Part model, mm, in its own coordinate system. A direction names the side the tool comes from. Give positions to 0.01 mm unless a question says otherwise; leave off trailing zeros. Write each loop counter-clockwise with the first axis right and the second up, starting at its lowest first coordinate (ties: lowest second). Pieces come first, ordered by that corner, then holes. Notation, with made-up numbers: M -9,70.5 L 41,70.5 A21 cw 41,81.5 Z; hole C 88,-14 d11. An arc over 180 degrees is marked long. Use CSV: the item, a comma, the result in double quotes. Start each with the question number.
1. Band-saw the part on D-D, the plane y = 63.5. List the corners of the cut face in (x, z).
2. Band-saw the part on C-C, the plane y = 74.5. List the corners of the cut face in (x, z), then the cut area to 3 significant figures.
3. Band-saw the part on B-B, the plane z = 37. List the corners of the cut face in (x, y).
4. Band-saw the part on A-A, the plane x = -37. List the corners of the cut face in (y, z), then the cut area to 3 significant figures.
5. Drop flat-ended pins along their axis: pin 1 Ø4 at (y, z) = (22.5, -35) entering from -X; pin 2 Ø3 at (x, y) = (-44.33, 38.65) entering from +Z; pin 3 Ø20 at (x, y) = (-61.65, 48.65) entering from -Z; pin 4 Ø1.5 at (x, z) = (21, 10) entering from -Y. Give the stop position or say it passes through.
6. 3-axis set-ups, long thin cutter, end or side, ignore diameter. For faces 5 (the face through (-22, 41, 1)), 6 (the face through (-52, 41, 6)), 7 (the face through (-56.574, 38.891, 7.014)): which of +Z, -Z, +X, -X, +Y, -Y reach the whole face in a straight line?
7. Drill centre lines: line 1 along Z through (x, y) = (10, 0.95) (3 decimals); line 2 along X through (y, z) = (0.9, -22) (3 decimals); line 3 along X through (y, z) = (48.65, -38.9). Where is each one in solid material? Low to high. Write a range as from..to.
8. Mould opens along Z. For faces 1 (the face through (-52, 48, -39.5)), 2 (the face through (0, 0, -1)), 3 (the face through (-52, 41, 8)), 4 (the face through (-52, 48, -37.5)) say: pulls with the +Z half, pulls with the -Z half, needs draft (parallel to the pull), parting line crosses it, or undercut.
from build123d import *

# Parameters (mm, degrees)
SKETCH_1_W                   = 50
SKETCH_1_H                   = 100
EXTRUDE_1_DEPTH              = 2
SKETCH_2_W                   = 3
SKETCH_2_H                   = 100
EXTRUDE_2_DEPTH              = 80
SKETCH_3_W                   = 2
SKETCH_3_H                   = 66.7
EXTRUDE_3_DEPTH              = 70
CUT_EXTRUDE_4_REACH          = 162.465
SKETCH_8_W                   = 2
SKETCH_8_H                   = 66.7
EXTRUDE_4_DEPTH              = 70
CUT_EXTRUDE_5_REACH          = 140.25
HOLE_WIZARD_M3_1_D           = 2.5
HOLE_WIZARD_M3_1_DEPTH       = 2
HOLE_WIZARD_M3_1_CSINK_D     = 3.05
HOLE_WIZARD_M3_1_CSINK_ANGLE = 90
FILLET_1_R                   = 2
CUT_EXTRUDE_6_REACH          = 140.25
SKETCH_12_R                  = 11
CUT_EXTRUDE_7_REACH          = 162.465
SKETCH_13_R                  = 14.5
SKETCH_14_W                  = 2
SKETCH_14_H                  = 66.7
EXTRUDE_5_DEPTH              = 70
CUT_EXTRUDE_8_REACH          = 156.14
SKETCH_15_R                  = 5.1
CUT_EXTRUDE_9_DEPTH          = 155.140358116
CUT_EXTRUDE_9_DEPTH_BACK     = 155.140358116
SKETCH_19_W                  = 2
SKETCH_19_H                  = 66.7
CUT_EXTRUDE_10_DEPTH         = 119.844436134
FILLET_2_R                   = 2
HOLE_WIZARD_M3_3_D           = 2.5
HOLE_WIZARD_M3_3_CSINK_D     = 3.05
HOLE_WIZARD_M3_3_CSINK_ANGLE = 90


# Read off the part's stored shape, not the designer's step: M1.6 螺纹孔1, M1.6 螺纹孔2
with BuildPart() as part:
    # 草图1 → 凸台-拉伸1 (new body)
    with BuildSketch(Plane(origin=(0, 0, 0), x_dir=(1, 0, 0), z_dir=(0, 1, 0))):
        Rectangle(SKETCH_1_W, SKETCH_1_H)
    extrude(amount=EXTRUDE_1_DEPTH)

    # 草图2 → 凸台-拉伸2 (add)
    with BuildSketch(Plane(origin=(0, 2, 0), x_dir=(1, 0, 0), z_dir=(0, 1, 0))):
        with Locations((-23.5, 0)):
            Rectangle(SKETCH_2_W, SKETCH_2_H)
    extrude(amount=EXTRUDE_2_DEPTH)

    # 草图3 → 凸台-拉伸3 (add)
    with BuildSketch(Plane.ZY.offset(25)):
        with Locations((-49, 48.65)):
            Rectangle(SKETCH_3_W, SKETCH_3_H)
    extrude(amount=EXTRUDE_3_DEPTH)

    # 草图4 → 切除-拉伸4 (cut, up to next)
    with BuildSketch(Plane(origin=(0, 0, -50), x_dir=(-1, 0, 0), z_dir=(0, 0, -1)), mode=Mode.PRIVATE) as cut_extrude_4_sk1:
        with BuildLine():
            Line((95, 82), (61.65, 82))
            ThreePointArc((61.65, 82), (85.232011153, 72.232011153), (95, 48.65))
            Line((95, 48.65), (95, 82))
        make_face()
    cut_extrude_4_tool1 = extrude(cut_extrude_4_sk1.sketch, amount=-CUT_EXTRUDE_4_REACH, mode=Mode.PRIVATE) & part.part
    # 草图4 → 切除-拉伸4 (cut, up to next)
    with BuildSketch(Plane(origin=(0, 0, -50), x_dir=(-1, 0, 0), z_dir=(0, 0, -1)), mode=Mode.PRIVATE) as cut_extrude_4_sk2:
        with BuildLine():
            ThreePointArc((95, 48.65), (85.232011153, 25.067988847), (61.65, 15.3))
            Line((61.65, 15.3), (95, 15.3))
            Line((95, 15.3), (95, 48.65))
        make_face()
    cut_extrude_4_tool2 = extrude(cut_extrude_4_sk2.sketch, amount=-CUT_EXTRUDE_4_REACH, mode=Mode.PRIVATE) & part.part
    add(cut_extrude_4_tool1.solids().sort_by_distance((-87.550679, 74.550679, -50))[0], mode=Mode.SUBTRACT)
    add(cut_extrude_4_tool2.solids().sort_by_distance((-87.550679, 22.749321, -50))[0], mode=Mode.SUBTRACT)

    # 草图8 → 凸台-拉伸4 (add)
    with BuildSketch(Plane.ZY.offset(25)):
        with Locations((7, 48.65)):
            Rectangle(SKETCH_8_W, SKETCH_8_H)
    extrude(amount=EXTRUDE_4_DEPTH)

    # 草图9 → 切除-拉伸5 (cut, up to next)
    with BuildSketch(Plane.XY.offset(8), mode=Mode.PRIVATE) as cut_extrude_5_sk1:
        with BuildLine():
            ThreePointArc((-95, 48.65), (-85.232011153, 72.232011153), (-61.65, 82))
            Line((-61.65, 82), (-95, 82))
            Line((-95, 82), (-95, 48.65))
        make_face()
    cut_extrude_5_tool1 = extrude(cut_extrude_5_sk1.sketch, amount=-CUT_EXTRUDE_5_REACH, mode=Mode.PRIVATE) & part.part
    # 草图9 → 切除-拉伸5 (cut, up to next)
    with BuildSketch(Plane.XY.offset(8), mode=Mode.PRIVATE) as cut_extrude_5_sk2:
        with BuildLine():
            ThreePointArc((-61.65, 15.3), (-85.232011153, 25.067988847), (-95, 48.65))
            Line((-95, 48.65), (-95, 15.3))
            Line((-95, 15.3), (-61.65, 15.3))
        make_face()
    cut_extrude_5_tool2 = extrude(cut_extrude_5_sk2.sketch, amount=-CUT_EXTRUDE_5_REACH, mode=Mode.PRIVATE) & part.part
    add(cut_extrude_5_tool1.solids().sort_by_distance((-87.550679, 74.550679, 8))[0], mode=Mode.SUBTRACT)
    add(cut_extrude_5_tool2.solids().sort_by_distance((-87.550679, 22.749321, 8))[0], mode=Mode.SUBTRACT)

    # M3 螺纹孔1
    with Locations(Plane.XY.offset(8)):
        with Locations((-78.970508076, 38.65), (-61.65, 68.65), (-44.329491924, 38.65)):
            CounterSinkHole(HOLE_WIZARD_M3_1_D / 2, HOLE_WIZARD_M3_1_CSINK_D / 2, depth=HOLE_WIZARD_M3_1_DEPTH, counter_sink_angle=HOLE_WIZARD_M3_1_CSINK_ANGLE)

    # 圆角1
    fillet_1_edges = [part.edges().sort_by_distance(p)[0] for p in [
        (-23.5, 82, 50),
        (25, 1, 50),
        (25, 1, -50),
    ]]
    fillet(fillet_1_edges, radius=FILLET_1_R)

    # 草图12 → 切除-拉伸6 (cut, up to next)
    with BuildSketch(Plane.XY.offset(8), mode=Mode.PRIVATE) as cut_extrude_6_sk1:
        with Locations((-61.65, 48.65)):
            Circle(SKETCH_12_R)
    cut_extrude_6_tool1 = extrude(cut_extrude_6_sk1.sketch, amount=-CUT_EXTRUDE_6_REACH, mode=Mode.PRIVATE) & part.part
    add(cut_extrude_6_tool1.solids().sort_by_distance((-61.65, 48.65, 8))[0], mode=Mode.SUBTRACT)

    # 草图13 → 切除-拉伸7 (cut, up to next)
    with BuildSketch(Plane(origin=(0, 0, -50), x_dir=(-1, 0, 0), z_dir=(0, 0, -1)), mode=Mode.PRIVATE) as cut_extrude_7_sk1:
        with Locations((61.65, 48.65)):
            Circle(SKETCH_13_R)
    cut_extrude_7_tool1 = extrude(cut_extrude_7_sk1.sketch, amount=-CUT_EXTRUDE_7_REACH, mode=Mode.PRIVATE) & part.part
    add(cut_extrude_7_tool1.solids().sort_by_distance((-61.65, 48.65, -50))[0], mode=Mode.SUBTRACT)

    # 草图14 → 凸台-拉伸5 (add)
    with BuildSketch(Plane.ZY.offset(25)):
        with Locations((-38.5, 48.65)):
            Rectangle(SKETCH_14_W, SKETCH_14_H)
    extrude(amount=EXTRUDE_5_DEPTH)

    # 草图15 → 切除-拉伸8 (cut, up to next)
    with BuildSketch(Plane(origin=(0, 0, -39.5), x_dir=(-1, 0, 0), z_dir=(0, 0, -1)), mode=Mode.PRIVATE) as cut_extrude_8_sk1:
        with Locations(Location((61.65, 48.65, 0), (0, 0, 90))):
            Circle(SKETCH_15_R)
    cut_extrude_8_tool1 = extrude(cut_extrude_8_sk1.sketch, amount=-CUT_EXTRUDE_8_REACH, mode=Mode.PRIVATE) & part.part
    add(cut_extrude_8_tool1.solids().sort_by_distance((-61.65, 48.65, -39.5))[0], mode=Mode.SUBTRACT)

    # 草图18 → 切除-拉伸9 (cut, two sides: drawn at the far end of the back side and taken through both)
    with BuildSketch(Plane(origin=(0, 0, -39.5), x_dir=(-1, 0, 0), z_dir=(0, 0, -1)).offset(-CUT_EXTRUDE_9_DEPTH_BACK)):
        with BuildLine():
            Line((95, 15.3), (95, 48.65))
            ThreePointArc((95, 48.65), (85.232011153, 25.067988847), (61.65, 15.3))
            Line((61.65, 15.3), (95, 15.3))
        make_face()
        with BuildLine():
            Line((95, 48.65), (95, 82))
            Line((95, 82), (61.65, 82))
            ThreePointArc((61.65, 82), (85.232011153, 72.232011153), (95, 48.65))
        make_face()
    extrude(amount=CUT_EXTRUDE_9_DEPTH + CUT_EXTRUDE_9_DEPTH_BACK, mode=Mode.SUBTRACT)

    # 草图19 → 切除-拉伸10 (cut, through all)
    with BuildSketch(Plane.ZY.offset(25)):
        with Locations((-49, 48.65)):
            Rectangle(SKETCH_19_W, SKETCH_19_H)
    extrude(amount=CUT_EXTRUDE_10_DEPTH, mode=Mode.SUBTRACT)

    # 圆角2
    fillet_2_edges = [part.edges().sort_by_distance(p)[0] for p in [
        (-23.5, 82, -50),
    ]]
    fillet(fillet_2_edges, radius=FILLET_2_R)

    # M3 螺纹孔3 (through all)
    with Locations(Plane(origin=(0, 2, 0), x_dir=(1, 0, 0), z_dir=(0, 1, 0))):
        with Locations((-2.7, 0), (21, 10), (21, -10)):
            CounterSinkHole(HOLE_WIZARD_M3_3_D / 2, HOLE_WIZARD_M3_3_CSINK_D / 2, counter_sink_angle=HOLE_WIZARD_M3_3_CSINK_ANGLE)

    # M1.6 螺纹孔1 outline → M1.6 螺纹孔1 (revolve, cut)
    with BuildSketch(Plane(origin=(10, 0, -28), x_dir=(1, 0, 0), z_dir=(0, 0, 1))):
        Polygon((0, 0), (0.625, 0), (0.625, 1.8), (0.825, 2), (0, 2), align=None)
    revolve(axis=Axis((10, 0, -28), (0, 1, 0)), mode=Mode.SUBTRACT)

    # Hole Wizard M1.6 _1 2 outline → Hole Wizard M1.6 _1 2 (revolve, cut)
    with BuildSketch(Plane(origin=(6.4, 0, -28), x_dir=(1, 0, 0), z_dir=(0, 0, 1))):
        Polygon((0, 0), (0.625, 0), (0.625, 1.8), (0.825, 2), (0, 2), align=None)
    revolve(axis=Axis((6.4, 0, -28), (0, 1, 0)), mode=Mode.SUBTRACT)

    # M1.6 螺纹孔2 outline → M1.6 螺纹孔2 (revolve, cut)
    with BuildSketch(Plane(origin=(10, 0, -22), x_dir=(1, 0, 0), z_dir=(0, 0, 1))):
        Polygon((0, 0), (0.625, 0), (0.625, 1.8), (0.825, 2), (0, 2), align=None)
    revolve(axis=Axis((10, 0, -22), (0, 1, 0)), mode=Mode.SUBTRACT)

    # Hole Wizard M1.6 _2 2 outline → Hole Wizard M1.6 _2 2 (revolve, cut)
    with BuildSketch(Plane(origin=(6.4, 0, -22), x_dir=(1, 0, 0), z_dir=(0, 0, 1))):
        Polygon((0, 0), (0.625, 0), (0.625, 1.8), (0.825, 2), (0, 2), align=None)
    revolve(axis=Axis((6.4, 0, -22), (0, 1, 0)), mode=Mode.SUBTRACT)


solid = part.part
Output:
1,outline,"M -91.51,-39.5 L -25,-39.5 L -25,-50 L -22,-50 L -22,50 L -25,50 L -25,8 L -91.51,8 L -91.51,6 L -25,6 L -25,-37.5 L -91.51,-37.5 Z"
2,outline,"M -82.72,-39.5 L -25,-39.5 L -25,-50 L -22,-50 L -22,50 L -25,50 L -25,8 L -82.72,8 L -82.72,6 L -25,6 L -25,-37.5 L -82.72,-37.5 Z"
2,area,"531 mm²"
3,outline,"M -25,0 L 25,0 L 25,2 L -22,2 L -22,82 L -25,82 Z"
4,outline,"M 15.3,-39.5 L 82,-39.5 L 82,-37.5 L 15.3,-37.5 Z; M 15.3,6 L 82,6 L 82,8 L 15.3,8 Z"
4,area,"267 mm²"
5,pin 1,"stops at x = -25"
5,pin 2,"stops at z = 7.98"
5,pin 3,"stops at z = -39.5"
5,pin 4,"passes through"
6,face 5,"+Z, -Z, +X, +Y"
6,face 6,"-X, +Y, -Y"
6,face 7,"+Z"
7,line 1,"z = -50..-28.625, -27.375..-22.625, -21.375..50"
7,line 2,"x = -25..5.775, 7.025..9.375, 10.625..25"
7,line 3,"x = -95..-66.75, -56.55..-22"
8,face 1,"pulls with the -Z half"
8,face 2,"needs draft"
8,face 3,"pulls with the +Z half"
8,face 4,"undercut"
